from build123d import *

# Parameters (mm, degrees)
F1_DEPTH  = 1524
F3_DEPTH  = 101.6
F5_D      = 6.5278
F5_DEPTH  = 12.7
F5_TIP    = 1.9611489744
F7_DEPTH  = 254
F9_D      = 6.5278
F9_DEPTH  = 101.6
F9_TIP    = 1.9611489744
F10_D     = 6.35
F12_D     = 2.9464
F12_DEPTH = 5.08
F12_TIP   = 0.885187864


with BuildPart() as f1:
    # F0 (on Front) → F1 (new body)
    with BuildSketch(Plane.XZ):
        with BuildLine():
            Line((0, -38.1), (0, 0))
            Line((0, 0), (0, 38.1))
            Line((0, 38.1), (-31.877, 38.1))
            Line((-31.877, 38.1), (-31.877, 35.56))
            ThreePointArc((-31.877, 35.56), (-30.0171280605, 31.0698719395), (-25.527, 29.21))
            Line((-25.527, 29.21), (-4.445, 29.21))
            Line((-4.445, 29.21), (-4.445, 0))
            Line((-4.445, 0), (-4.445, -29.21))
            Line((-4.445, -29.21), (-25.527, -29.21))
            ThreePointArc((-25.527, -29.21), (-30.0171280605, -31.0698719395), (-31.877, -35.56))
            Line((-31.877, -35.56), (-31.877, -38.1))
            Line((-31.877, -38.1), (0, -38.1))
        make_face()
        with BuildLine():
            Line((0, 38.1), (0, 0))
            Line((0, 0), (4.445, 0))
            Line((4.445, 0), (4.445, 29.21))
            Line((4.445, 29.21), (25.527, 29.21))
            ThreePointArc((25.527, 29.21), (30.0171280605, 31.0698719395), (31.877, 35.56))
            Line((31.877, 35.56), (31.877, 38.1))
            Line((31.877, 38.1), (0, 38.1))
        make_face()
        with BuildLine():
            Line((4.445, 0), (0, 0))
            Line((0, 0), (0, -38.1))
            Line((0, -38.1), (31.877, -38.1))
            Line((31.877, -38.1), (31.877, -35.56))
            ThreePointArc((31.877, -35.56), (30.0171280605, -31.0698719395), (25.527, -29.21))
            Line((25.527, -29.21), (4.445, -29.21))
            Line((4.445, -29.21), (4.445, 0))
        make_face()
    extrude(amount=F1_DEPTH)

    # F2 (on face) → F3 (cut)
    with BuildSketch(Plane.XY.offset(38.1)):
        with BuildLine():
            ThreePointArc((-31.877, 0), (-19.0959593861, -15.3024519653), (0, -21.03519742))
            Line((0, -21.03519742), (0, 0))
            Line((0, 0), (-31.877, 0))
        make_face()
        with BuildLine():
            Line((0, 0), (0, -21.03519742))
            ThreePointArc((0, -21.03519742), (24.5160992105, -10.8802966305), (34.671, 13.63580258))
            ThreePointArc((34.671, 13.63580258), (-6.9595536495, 47.6011209798), (-31.877, 0))
            Line((-31.877, 0), (0, 0))
        make_face()
    extrude(amount=-F3_DEPTH, mode=Mode.SUBTRACT)

    # F5
    with Locations(Plane.XY.offset(38.1)):
        with Locations((-15.875, -182.96019742), (15.875, -163.91019742), (15.875, -182.96019742), (-15.875, -163.91019742)):
            Hole(F5_D / 2, depth=F5_DEPTH)
            with Locations((0, 0, -(F5_DEPTH + F5_TIP / 2))):  # 118° drill point
                Cone(0, F5_D / 2, F5_TIP, mode=Mode.SUBTRACT)

    # F6 (on Front) → F7 (cut)
    with BuildSketch(Plane.XZ):
        Polygon((40.005, -29.21), (4.445, -29.21), (-4.445, -29.21), (-40.005, -29.21), (-40.005, -38.1), (40.005, -38.1), align=None)
    extrude(amount=F7_DEPTH, mode=Mode.SUBTRACT)

    # F9
    with Locations(Plane.XY.offset(38.1)):
        with Locations((-19.05, -1428.75), (-19.05, -1447.8), (-19.05, -1466.85), (-19.05, -1485.9), (-19.05, -1504.95), (19.05, -1504.95), (19.05, -1485.9), (19.05, -1466.85), (19.05, -1447.8), (19.05, -1428.75)):
            Hole(F9_D / 2, depth=F9_DEPTH)
            with Locations((0, 0, -(F9_DEPTH + F9_TIP / 2))):  # 118° drill point
                Cone(0, F9_D / 2, F9_TIP, mode=Mode.SUBTRACT)

    # F10 (through all)
    with Locations(Plane.XY.offset(38.1)):
        with Locations((19.05, -1377.55376), (19.05, -1358.61298), (-19.05, -1358.61298), (-19.05, -1377.55376)):
            Hole(F10_D / 2)

    # F12
    with Locations(Plane.XY.offset(38.1)):
        with Locations((27.64536, -1099.47964), (27.64536, -1130.3), (0, -1099.47964), (-27.64536, -1099.47964), (-27.64536, -1130.3), (-27.64536, -1161.12036), (0, -1161.12036), (27.64536, -1161.12036)):
            Hole(F12_D / 2, depth=F12_DEPTH)
            with Locations((0, 0, -(F12_DEPTH + F12_TIP / 2))):  # 118° drill point
                Cone(0, F12_D / 2, F12_TIP, mode=Mode.SUBTRACT)


solid = f1.part
Here's how the part is built. I have some questions about the finished solid (model axes, mm). A direction names the side the tool comes from. Coordinates: 2 decimals unless noted, no trailing zeros. Order: outer loops, then holes, each group sorted by start corner. A loop starts at its lowest first (then second) coordinate and runs counter-clockwise, first axis right, second up. Notation, with made-up numbers: (54, 75.25) -> (60, 75.25) arc R23 ccw to (60, 112.25) -> close; hole circle Ø10 at (48.5, -22). An arc over 180 degrees is marked (long way). Answer in a Markdown table with one row per item.
(1) Thinking about a two-plate mould opening in Z: for faces 3 (the face through (4.445, -762, 0)), 4 (the face through (0, -751, 38.1)), 5 (the face through (0, -880, -38.1)), which applies, +Z half, -Z half, draft (parallel to the pull), parting line (faces both ways), or undercut?
Answer key:
| item | result |
|---|---|
| face 3 | undercut |
| face 4 | +Z half |
| face 5 | -Z half |
(2) On a 3-axis mill with a long thin cutter (end or side, diameter ignored), from which of +Z, -Z, +X, -X, +Y, -Y can I reach the whole of each face in a straight line? I mean faces 1 (the face through (0, -1524, 3)), 2 (the face through (-4.445, -762, 0)). Say none if no direction works.
Answer key:
| item | result |
|---|---|
| face 1 | +Z, -Z, +X, -X, -Y |
| face 2 | -X, +Y, -Y |
(3) I want a section at A-A on y = -1234. List the corners of the cut face in (x, z) for me (3 decimals).
Answer key:
| item | result |
|---|---|
| outline | (-31.877, -38.1) -> (31.877, -38.1) -> (31.877, -35.56) arc R6.35 ccw to (25.527, -29.21) -> (4.445, -29.21) -> (4.445, 29.21) -> (25.527, 29.21) arc R6.35 ccw to (31.877, 35.56) -> (31.877, 38.1) -> (-31.877, 38.1) -> (-31.877, 35.56) arc R6.35 ccw to (-25.527, 29.21) -> (-4.445, 29.21) -> (-4.445, -29.21) -> (-25.527, -29.21) arc R6.35 ccw to (-31.877, -35.56) -> close |
(4) Please list where these lines run through material, in increasing order: probe 1 along Y at (x, z) = (0, 35.75); probe 2 along Z at (x, y) = (-10, -1422.5); probe 3 along X at (y, z) = (-1428, -32).
Answer key:
| item | result |
|---|---|
| probe 1 | -1524 to -1162.59, -1159.65 to -1100.95, -1098.01 to -21.04 |
| probe 2 | -38.1 to -29.21, 29.21 to 38.1 |
| probe 3 | -30.79 to -22.23, -15.87 to 15.87, 22.23 to 30.79 |
(5) I want a section at B-B on z = 17. List the corners of the cut face in (x, y) for me (3 decimals).
Answer key:
| item | result |
|---|---|
| outline | (-4.445, -1524) -> (4.445, -1524) -> (4.445, -20.749) arc R34.671 cw to (-4.445, -20.749) -> close |
(6) Will these pins go through, and if not, where does the flat tip stop? pin 1 Ø2.5 at (x, y) = (0, -195.5) entering from -Z; pin 2 Ø12 at (y, z) = (-655, 22) entering from -X (3 decimals).
Answer key:
| item | result |
|---|---|
| pin 1 | z = -29.21 |
| pin 2 | x = -4.445 |
(7) I want a section at C-C on y = -234. List the corners of the cut face in (x, z) for me (3 decimals), then the cut area to 3 significant figures.
Answer key:
| item | result |
|---|---|
| outline | (-31.877, 35.56) arc R6.35 ccw to (-25.527, 29.21) -> (-4.445, 29.21) -> (-4.445, -29.21) -> (4.445, -29.21) -> (4.445, 29.21) -> (25.527, 29.21) arc R6.35 ccw to (31.877, 35.56) -> (31.877, 38.1) -> (-31.877, 38.1) -> close |
| area | 1,070 mm^2 |
